For this review, take the finished solid that the model builds, in its own axes (mm). Give positions to 0.01 mm unless a question says otherwise; leave off trailing zeros. Order: outer loops, then holes, each group sorted by start corner. A loop starts at its lowest first (then second) coordinate and runs counter-clockwise, first axis right, second up.
Item 1: For P1, Ø1.5, axis at y = -108.5, z = -55.5, coming from the -X side; P2, Ø10, axis at y = -154, z = -59.5, coming from the -X side; P3, Ø1, axis at x = -74, y = -461, coming from the -Z side, all flat-tipped, find the tip position at first contact; note any pin that passes through.
Item 2: Consider section D-D (y = -631). Give the boundary of the cut face in (x, z).
Item 3: Consider section B-B (x = -83). Give the boundary of the cut face in (y, z).
Item 4: For probe 1 along X at (y, z) = (-602, 23.5); probe 2 along Z at (x, y) = (-116, -66.5); probe 3 along X at (y, z) = (-116, -45.5), list the stretches that pass through material, from the lowest coordinate up.
Item 5: Consider section A-A (y = -273). Give the boundary of the cut face in (x, z).
Item 6: Consider section C-C (z = 49). Give the boundary of the cut face in (x, y).
```python
from build123d import *

# Parameters (mm, degrees)
F1_DEPTH    = 762
F2_T1_DEPTH = 1300.1781500313
F2_T3_DEPTH = 1300.1781500313
F2_T5_DEPTH = 1300.1781500313
F2_T7_DEPTH = 1300.1781500313


# Not quite as in the source:
# - a fillet or chamfer that OpenCascade refuses, or shapes differently, is made with other operations: its cross-section is extruded or revolved along the edge and cut away or added


with BuildPart() as f1:
    # F0 (on Front) → F1 (new body)
    with BuildSketch(Plane.XZ):
        Polygon((25.4, 76.2), (0, 76.2), (-25.4, 76.2), (-127.5811195374, 25.4), (-127.5811195374, 0), (-127.5811195374, -25.4), (-25.4, -76.2), (0, -76.2), (25.4, -76.2), (127.5811195374, -25.4), (127.5811195374, 0), (127.5811195374, 25.4), align=None)
    extrude(amount=F1_DEPTH)

    # F2: chamfer of 228.6 x 83.2035955533 on 4 edges, made by hand

    # F2_s2 → F2_t1 (cut)
    with BuildSketch(Plane(origin=(541.036756959, 0, 268.9798993978), x_dir=(0, 1, 0), z_dir=(-0.8954433759, 0, -0.4451754267))):
        Polygon((-762, 3.6633544712), (-533.4, -79.540241082), (-762, -79.540241082), align=None)
    extrude(amount=F2_T1_DEPTH, mode=Mode.SUBTRACT)

    # F2_s4 → F2_t3 (cut)
    with BuildSketch(Plane(origin=(623.1991549624, 0, -309.8274633849), x_dir=(0, 1, 0), z_dir=(-0.8954433759, 0, 0.4451754267))):
        Polygon((-533.4, -79.540241082), (-762, 3.6633544712), (-762, -79.540241082), align=None)
    extrude(amount=F2_T3_DEPTH, mode=Mode.SUBTRACT)

    # F2_s6 → F2_t5 (cut)
    with BuildSketch(Plane(origin=(-541.036756959, 0, -268.9798993978), x_dir=(0, 1, 0), z_dir=(0.8954433759, 0, 0.4451754267))):
        Polygon((-762, 3.6633544712), (-533.4, -79.540241082), (-762, -79.540241082), align=None)
    extrude(amount=F2_T5_DEPTH, mode=Mode.SUBTRACT)

    # F2_s8 → F2_t7 (cut)
    with BuildSketch(Plane(origin=(-623.1991549624, 0, 309.8274633849), x_dir=(0, 1, 0), z_dir=(0.8954433759, 0, -0.4451754267))):
        Polygon((-762, 3.6633544712), (-533.4, -79.540241082), (-762, -79.540241082), align=None)
    extrude(amount=F2_T7_DEPTH, mode=Mode.SUBTRACT)


solid = f1.part
```
Resolved:
1. P1: stops at x = -68.55
1. P2: stops at x = -69.05
1. P3: stops at z = -52.29
2. outline: (-98.88, 0) - (0, -49.16) - (98.88, 0) - (0, 49.16) - close
3. outline: (-650.42, 0) - (-533.4, -47.56) - (0, -47.56) - (0, 47.56) - (-533.4, 47.56) - close
4. probe 1: x = -75.32 to 75.32
4. probe 2: z = -31.16 to 31.16
4. probe 3: x = -87.15 to 87.15
5. outline: (-127.58, -25.4) - (-25.4, -76.2) - (25.4, -76.2) - (127.58, -25.4) - (127.58, 25.4) - (25.4, 76.2) - (-25.4, 76.2) - (-127.58, 25.4) - close
6. outline: (-80.11, -533.4) - (0, -631.38) - (80.11, -533.4) - (80.11, 0) - (-80.11, 0) - close
